```python
from build123d import *

# Parameters (mm, degrees)
BOSS_EXTRUDE1_DEPTH = 18
SKETCH2_W           = 15
SKETCH2_H           = 14
CUT_EXTRUDE1_DEPTH  = 15
CUT_EXTRUDE2_START  = -3.742641
SKETCH7_W           = 2
SKETCH7_H           = 3
CUT_EXTRUDE2_DEPTH  = 3.242641
CUT_EXTRUDE4_REACH  = 30.583
SKETCH9_W           = 1
SKETCH9_H           = 6
BOSS_EXTRUDE2_DEPTH = 3
CUT_EXTRUDE5_REACH  = 30.583
SKETCH11_W          = 1
SKETCH11_H          = 6
BOSS_EXTRUDE3_DEPTH = 3
CUT_EXTRUDE6_DEPTH  = 4
SKETCH13_W          = 1
SKETCH13_H          = 6
BOSS_EXTRUDE4_DEPTH = 2.5
SKETCH14_W          = 1
SKETCH14_H          = 8
BOSS_EXTRUDE5_DEPTH = 0.5
FILLET3_R           = 1
FILLET4_R           = 0.5


with BuildPart() as part:
    # Sketch1 → Boss-Extrude1 (new body)
    with BuildSketch(Plane(origin=(0, 0, 0), x_dir=(1, 0, 0), z_dir=(0, 1, 0))):
        Polygon((0, 0), (0, 18), (3, 18), (18, 3), (18, 0), align=None)
    extrude(amount=BOSS_EXTRUDE1_DEPTH)

    # Sketch2 → Cut-Extrude1 (cut)
    with BuildSketch(Plane(origin=(0, 0, -18), x_dir=(-1, 0, 0), z_dir=(0, 0, -1))):
        with Locations((-10.5, 9)):
            Rectangle(SKETCH2_W, SKETCH2_H)
    extrude(amount=-CUT_EXTRUDE1_DEPTH, mode=Mode.SUBTRACT)

    # Sketch3 → Cut-Loft1 section 0
    with BuildSketch(Plane(origin=(0, 0, -3), x_dir=(-1, 0, 0), z_dir=(0, 0, -1))):
        with BuildLine():
            Line((-15, 11.5), (-9, 11.5))
            Line((-9, 11.5), (-9, 6.5))
            Line((-9, 6.5), (-15, 6.5))
            Line((-15, 6.5), (-15, 11.5))
        make_face()
    # Sketch6 → Cut-Loft1 section 1
    with BuildSketch(Plane.XY):
        with BuildLine():
            Line((15, 11.5), (5, 11.5))
            Line((5, 11.5), (5, 6.5))
            Line((5, 6.5), (15, 6.5))
            Line((15, 6.5), (15, 11.5))
        make_face()
    loft(mode=Mode.SUBTRACT)

    # Sketch4 → Cut-Loft2 section 0
    with BuildSketch(Plane(origin=(3, 0, 0), x_dir=(0, 0, -1), z_dir=(1, 0, 0))):
        with BuildLine():
            Line((9, 11.5), (15, 11.5))
            Line((15, 11.5), (15, 6.5))
            Line((15, 6.5), (9, 6.5))
            Line((9, 6.5), (9, 11.5))
        make_face()
    # Sketch5 → Cut-Loft2 section 1
    with BuildSketch(Plane.ZY):
        with BuildLine():
            Line((-15, 11.5), (-5, 11.5))
            Line((-5, 11.5), (-5, 6.5))
            Line((-5, 6.5), (-15, 6.5))
            Line((-15, 6.5), (-15, 11.5))
        make_face()
    loft(mode=Mode.SUBTRACT)

    # Sketch7 → Cut-Extrude2 (cut)
    with BuildSketch(Plane(origin=(10.5, 0, -10.5), x_dir=(-0.7071067811865475, 0, -0.7071067811865477), z_dir=(0.7071067811865477, 0, -0.7071067811865475)).offset(CUT_EXTRUDE2_START)):
        with Locations((12.106601718, 14.5)):
            Rectangle(SKETCH7_W, SKETCH7_H)
        with Locations((12.106601718, 3.5)):
            Rectangle(SKETCH7_W, SKETCH7_H)
        with Locations((-12.106601718, 14.5)):
            Rectangle(SKETCH7_W, SKETCH7_H)
        with Locations((-12.106601718, 3.5)):
            Rectangle(SKETCH7_W, SKETCH7_H)
    extrude(amount=CUT_EXTRUDE2_DEPTH, mode=Mode.SUBTRACT)

    # Cut-Extrude4: up to this face of the body (flat: up to its plane)
    cut_extrude4_end = Plane(part.part.faces().sort_by_distance((0.76429774, 13, -17.23570226))[0])
    # Sketch8 → Cut-Extrude4 (cut, up to the picked face)
    with BuildSketch(Plane.XZ.offset(-5), mode=Mode.PRIVATE) as cut_extrude4_sk1:
        Polygon((0.707163247, -18), (2.207135014, -16.500028233), (-0.113993924, -14.178899295), (-1.613965691, -15.678871062), align=None)
    cut_extrude4_tool1 = split(extrude(cut_extrude4_sk1.sketch, amount=-CUT_EXTRUDE4_REACH, mode=Mode.PRIVATE), bisect_by=cut_extrude4_end, keep=Keep.BOTH, mode=Mode.PRIVATE)
    add(cut_extrude4_tool1.solids().sort_by(Axis((0.296585, 5, -16.08945), (0, 1, 0)))[0], mode=Mode.SUBTRACT)


with BuildPart() as cut_extrude4_kept_piece:
    # of the separate pieces the step leaves, the one the design keeps (cut_extrude4_pieces_kept)
    add(part.part.solids().sort_by_distance((0, 0, 0))[0])

    # Sketch9 → Boss-Extrude2 (add)
    with BuildSketch(Plane(origin=(9.353581623, 0, -9.353581623), x_dir=(0.7071067811865475, 0, 0.7071067811865477), z_dir=(-0.7071067811865477, 0, 0.7071067811865475))):
        with Locations((-11.477882134, 9)):
            Rectangle(SKETCH9_W, SKETCH9_H)
    extrude(amount=BOSS_EXTRUDE2_DEPTH)

    # Cut-Extrude5: up to this face of the body (flat: up to its plane)
    cut_extrude5_end = Plane(cut_extrude4_kept_piece.part.faces().sort_by_distance((17.23570226, 5, -0.76429774))[0])
    # Sketch10 → Cut-Extrude5 (cut, up to the picked face)
    with BuildSketch(Plane(origin=(0, 13, 0), x_dir=(1, 0, 0), z_dir=(0, 1, 0)), mode=Mode.PRIVATE) as cut_extrude5_sk1:
        Polygon((18.647815387, 0.23086427), (16.585786438, 2.292893219), (13.714418547, -0.578474672), (15.776447496, -2.640503621), align=None)
    cut_extrude5_tool1 = split(extrude(cut_extrude5_sk1.sketch, amount=-CUT_EXTRUDE5_REACH, mode=Mode.PRIVATE), bisect_by=cut_extrude5_end, keep=Keep.BOTH, mode=Mode.PRIVATE)
    add(cut_extrude5_tool1.solids().sort_by(Axis((16.181117, 13, 0.173805), (0, -1, 0)))[0], mode=Mode.SUBTRACT)

    # Sketch11 → Boss-Extrude3 (add)
    with BuildSketch(Plane(origin=(9.439339828, 0, -9.439339828), x_dir=(0.7071067811865474, 0, 0.7071067811865478), z_dir=(-0.7071067811865478, 0, 0.7071067811865474))):
        with Locations((11.356601718, 9)):
            Rectangle(SKETCH11_W, SKETCH11_H)
    extrude(amount=BOSS_EXTRUDE3_DEPTH)

    # Sketch12 → Cut-Extrude6 (cut, symmetric)
    with BuildSketch(Plane(origin=(0, 9, 0), x_dir=(1, 0, 0), z_dir=(0, 1, 0))):
        Polygon((0, 3), (0, 0), (3, 0), align=None)
    extrude(amount=CUT_EXTRUDE6_DEPTH, both=True, mode=Mode.SUBTRACT)

    # Sketch13 → Boss-Extrude4 (add)
    with BuildSketch(Plane(origin=(1.5, 0, -1.5), x_dir=(0.7071067811865475, 0, 0.7071067811865477), z_dir=(-0.7071067811865477, 0, 0.7071067811865475))):
        with Locations((1.621320344, 9)):
            Rectangle(SKETCH13_W, SKETCH13_H)
        with Locations((-1.621320344, 9)):
            Rectangle(SKETCH13_W, SKETCH13_H)
    extrude(amount=BOSS_EXTRUDE4_DEPTH)

    # Sketch14 → Boss-Extrude5 (add, symmetric)
    with BuildSketch(Plane(origin=(1.5, 0, -1.5), x_dir=(0.7071067811865475, 0, 0.7071067811865477), z_dir=(-0.7071067811865477, 0, 0.7071067811865475))):
        with Locations((0, 9)):
            Rectangle(SKETCH14_W, SKETCH14_H)
    extrude(amount=BOSS_EXTRUDE5_DEPTH, both=True)

    # Fillet3
    fillet3_edges = [cut_extrude4_kept_piece.edges().sort_by_distance(p)[0] for p in [
        (-1.237380402, 9, -15.701902961),
        (-1.767766953, 9, -1.232233047),
        (1.232233047, 9, 1.767766953),
        (15.701902961, 9, 1.065863992),
        (0, 1, -18),
        (0, 17, -18),
        (1.5, 18, -18),
        (1.5, 0, -18),
        (9, 0, 0),
        (18, 0, -1.5),
        (10.5, 0, -10.5),
        (9, 18, 0),
        (18, 18, -1.5),
        (10.5, 18, -10.5),
        (0, 18, -9),
        (0, 0, -9),
        (0, 15.5, 0),
        (0, 2.5, 0),
    ]]
    fillet(fillet3_edges, radius=FILLET3_R - 0.0001)  # a hair under: the kernel refuses the full size

    # Fillet4
    fillet4_edges = [cut_extrude4_kept_piece.edges().sort_by_distance(p)[0] for p in [
        (15.70710656, 14.5, 2.21e-07),
        (15.70710656, 3.5, 2.21e-07),
        (5, 9, 0),
        (9.646446609, 6.5, 0),
        (0, 9, -5),
        (9.646446609, 11.5, 0),
        (0, 6.5, -9.646446609),
        (0, 11.5, -9.646446609),
        (-2.21e-07, 14.5, -15.70710656),
        (-2.21e-07, 3.5, -15.70710656),
    ]]
    fillet(fillet4_edges, radius=FILLET4_R)


solid = cut_extrude4_kept_piece.part
```
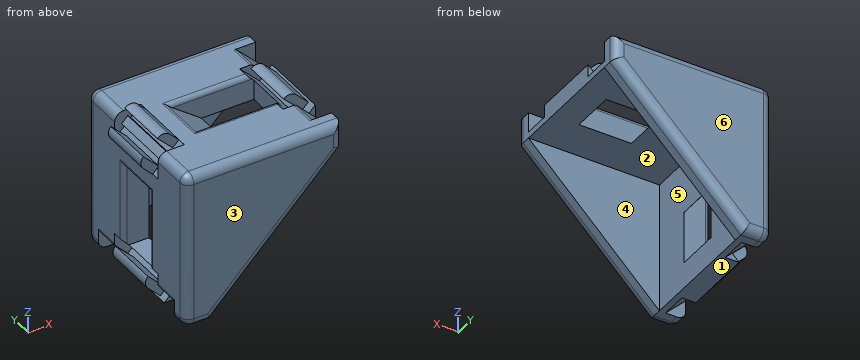
For this review, take the finished solid that the model builds, in its own axes (mm). Face numbers are marked on the shaded views. A direction names the side the tool comes from. Coordinates: 2 decimals unless noted, no trailing zeros. Write each loop counter-clockwise with the first axis right and the second up, starting at its lowest first coordinate (ties: lowest second). Pieces come first, ordered by that corner, then holes. Notation, with made-up numbers: (-37.75, -40) - (13.25, -40) arc R37 ccw to (13.25, -3) - close; hole circle Ø11 at (-14.5, -2.75). An arc over 180 degrees is marked (long way). Answer in a Markdown table with one row per item. Add a question column.
Q1. Draft analysis for pull direction Y (two halves, no side actions). For the marked faces 1, 2, 3 and 4, state which applies: +Y half, -Y half, draft (parallel to the pull), parting line (faces both ways), or undercut.
Q2. For P1, Ø5, axis at x = 14, z = -11, coming from the -Y side; P2, Ø2.5, axis at x = 1.5, z = 0.5, coming from the +Y side; P3, Ø1.5, axis at y = 15, z = -5.5, coming from the +X side; P4, Ø0.8, axis at x = 17.5, z = -1.5, coming from the -Y side (3 decimals), all flat-tipped, find the tip position at first contact; note any pin that passes through.
Q3. We need section A-A, the plane y = 16.5. State the section outline as (x, z) points.
Q4. Tool access review of the marked faces 5 and 6: name each direction out of +Z, -Z, +X, -X, +Y, -Y from which nothing blocks a thin tool from reaching the whole face with its end or side.
Q5. For probe 1 along Y at (x, z) = (4, -6); probe 2 along X at (y, z) = (13, -13.5); probe 3 along Z at (x, y) = (14.25, 2.75), list the stretches that pass through material, from the lowest coordinate up.
Answer list:
| question | item | result |
|---|---|---|
| 1 | face 1 | draft |
| 1 | face 2 | undercut |
| 1 | face 3 | -Y half |
| 1 | face 4 | undercut |
| 2 | P1 | passes through |
| 2 | P2 | stops at y = 17.97 |
| 2 | P3 | stops at x = 3 |
| 2 | P4 | stops at y = 0.005 |
| 3 | outline | (0, -17) arc R1 ccw to (1, -18) - (3, -18) - (18, -3) - (18, 0) - (1, 0) arc R1 ccw to (0, -1) - close |
| 4 | face 5 | -Z, +X |
| 4 | face 6 | +Z, -Z, +X, -X, +Y |
| 5 | probe 1 | y = 0 to 2, 16 to 18 |
| 5 | probe 2 | x = 0 to 3 |
| 5 | probe 3 | z = -3 to 0 |
